Model file for the job. Use its own axes, mm. Give positions to 0.01 mm unless a question says otherwise; leave off trailing zeros. Loops run counter-clockwise (first coordinate to the right, second up) from the corner with the lowest first, then second, coordinate; pieces in that order, holes last. Notation, with made-up numbers: M -4,69.5 L 1,69.5 A20 cw 1,104.5 Z; hole C 56,6 d8. An arc over 180 degrees is marked long. Answer in a Markdown table with one row per item.
Autodesk Inventor part; units mm, degrees
ref_plane "YZ Plane" through (0, 0, 0) normal (1, 0, 0) x (0, 1, 0)
ref_plane "XZ Plane" through (0, 0, 0) normal (0, 1, 0) x (-1, 0, 0)
ref_plane "XY Plane" through (0, 0, 0) normal (0, 0, 1) x (1, 0, 0)
sketch "草圖1" plane through (0, 0, 0) normal (0, 0, 1) x (1, 0, 0)
  line L0 (-140, 0) -> (140, 0) construction
  line L1 (-140, 0) -> (140, 0) construction
  line L2 (-140, -9) -> (140, -9)
  line L3 (140, 9) -> (-140, 9)
  arc A0 (-140, 9) -> (-140, -9) centre (-140, 0) ccw
  arc A1 (140, -9) -> (140, 9) centre (140, 0) ccw
  line L4 (-140, -2.35) -> (140, -2.35) construction
  line L5 (-140, -4.5) -> (140, -4.5)
  line L6 (140, -0.2) -> (-140, -0.2)
  arc A2 (-140, -0.2) -> (-140, -4.5) centre (-140, -2.35) ccw
  arc A3 (140, -4.5) -> (140, -0.2) centre (140, -2.35) ccw
  line L7 (140, -2.35) -> (140, 0) construction
  line L8 (-140, 9) -> (-149, 9)
  line L9 (-149, 9) -> (-149, -9)
  line L10 (-149, -9) -> (-140, -9)
  line L11 (-140, -9) -> (-140, 9)
  line L12 (140, 9) -> (149, 9)
  line L13 (149, 9) -> (149, -9)
  line L14 (149, -9) -> (140, -9)
  line L15 (140, -9) -> (140, 9)
  point P0 (0, 0)
  point P1 (0, 0)
  point P2 (0, 0)
  point P3 (0, -2.35)
  point P4 (149, 0)
  point P5 (-140, -9)
  point P6 (-149, 0)
  dimension "d5" = 9
  dimension "d7" = 280
  dimension "d22" = 2.15
  dimension "d24" = 4.5
extrude "擠出1" add sketch "草圖1" along normal blind 3 contours L11 L5 L15 L2 | L10 L9 A0 | A0 L11 A2 | L15 A3 A1 | A1 L13 L14 | L9 L8 A0 | A1 L12 L13 | L3 L15 L6 L11
sketch "草圖2" plane through (0, 0, 3) normal (0, 0, 1) x (1, 0, 0)
  line L0 (-208.6, 0) -> (208.6, 0)
  line L1 (-130, -9) -> (-122, -9)
  line L2 (-122, -9) -> (-122, -12)
  line L3 (-122, -12) -> (-130, -12)
  line L4 (-130, -12) -> (-130, -9)
  line L5 (122, -9) -> (130, -9)
  line L6 (130, -9) -> (130, -12)
  line L7 (130, -12) -> (122, -12)
  line L8 (122, -12) -> (122, -9)
  arc A0 (-140, -0.2) -> (-140, -4.5) centre (-140, -2.35) ccw
  arc A1 (140, -4.5) -> (140, -0.2) centre (140, -2.35) ccw
  line L9 (-149, -9) -> (149, -9)
  point P0 (0, 0)
  point P1 (130, -10.5)
  point P2 (-130, -10.5)
  dimension "d17" = 8
  dimension "d18" = 3
  dimension "d19" = 3
  dimension "d20" = 8
  dimension "d25" = 10
  dimension "d26" = 10
extrude "擠出2" add sketch "草圖2" against normal up to surface (3 mm away)
ref_plane "工作平面2" through (-140, -2.35, 0) normal (0, 1, 0) x (1, 0, 0)
sketch "草圖4" plane through (0, 0, 3) normal (0, 0, 1) x (1, 0, 0)
  line L0 (149, 9) -> (-149, 9)
  line L1 (-149, -9) -> (-130, -9)
  line L2 (-149, 9) -> (-146, 9)
  line L3 (-146, 9) -> (-146, -9)
  line L4 (-146, -9) -> (-149, -9)
  line L5 (-149, -9) -> (-149, 9)
  line L6 (-149, 9) -> (-149, -9)
  line L7 (-149, 3) -> (-146, 3)
  line L8 (-146, 3) -> (-146, -3)
  line L9 (-146, -3) -> (-149, -3)
  line L10 (-149, -3) -> (-149, 3)
  line L11 (149, -9) -> (149, 9)
  line L12 (149, -9) -> (146, -9)
  line L13 (146, -9) -> (146, 9)
  line L14 (146, 9) -> (149, 9)
  line L15 (149, 9) -> (149, -9)
  line L16 (149, -3) -> (146, -3)
  line L17 (146, -3) -> (146, 3)
  line L18 (146, 3) -> (149, 3)
  line L19 (149, 3) -> (149, -3)
  point P0 (0, 0)
  dimension "d27" = 6
  dimension "d28" = 6
  dimension "d29" = 3
  dimension "d32" = 3
extrude "擠出3" cut sketch "草圖4" against normal up to surface (3 mm away) contours L11 L18 L13 L0 | L3 L7 L5 L0 | L11 L12 L13 L16 | L3 L1 L5 L9
sketch "草圖5" plane through (0, 0, 3) normal (0, 0, 1) x (1, 0, 0)
  arc A0 (-140, -0.2) -> (-140, -4.5) centre (-140, -2.35) ccw
  line L0 (-140, -0.2) -> (140, -0.2)
  arc A1 (140, -4.5) -> (140, -0.2) centre (140, -2.35) ccw
  line L1 (140, -4.5) -> (-140, -4.5)
  line L2 (-146, 9) -> (-146, 3)
  line L3 (-146, 3) -> (-149, 3)
  line L4 (-149, 3) -> (-149, -3)
  line L5 (-149, -3) -> (-146, -3)
  line L6 (-146, -3) -> (-146, -9)
  line L7 (-146, -9) -> (-130, -9)
  line L8 (-130, -9) -> (-130, -12)
  line L9 (-130, -12) -> (-122, -12)
  line L10 (-122, -12) -> (-122, -9)
  line L11 (-122, -9) -> (122, -9)
  line L12 (122, -9) -> (122, -12)
  line L13 (122, -12) -> (130, -12)
  line L14 (130, -12) -> (130, -9)
  line L15 (130, -9) -> (146, -9)
  line L16 (146, -9) -> (146, -3)
  line L17 (146, -3) -> (149, -3)
  line L18 (149, -3) -> (149, 3)
  line L19 (149, 3) -> (146, 3)
  line L20 (146, 3) -> (146, 9)
  line L21 (146, 9) -> (-146, 9)
  point P0 (0, 0)
equation "\"d32\" = d29"
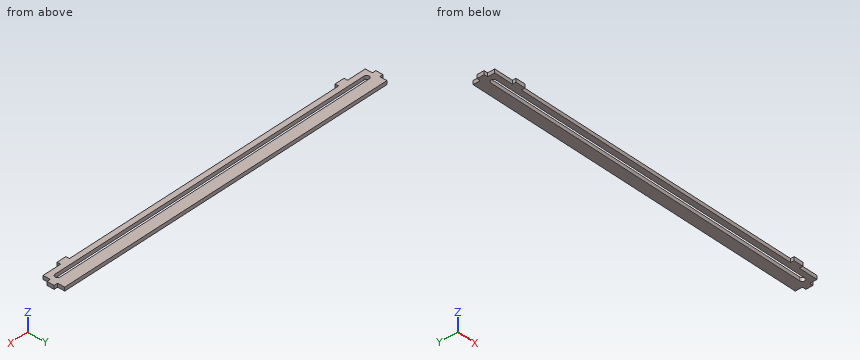
(1) Saw through at A-A, the plane x = -127.5. Give the cut face in (y, z).
Established:
| item | result |
|---|---|
| outline | M -12,0 L -4.5,0 L -4.5,3 L -12,3 Z; M -0.2,0 L 9,0 L 9,3 L -0.2,3 Z |
(2) Flat gauge pins, fed straight in: P1, Ø0.9, axis at y = 5.5, z = 2, coming from the +X side; P2, Ø1.5, axis at x = 147, z = 1, coming from the +Y side; P3, Ø0.9, axis at y = -10, z = 2, coming from the +X side. Where does each tip first touch, or does it go through?
Established:
| item | result |
|---|---|
| P1 | stops at x = 146 |
| P2 | stops at y = 3 |
| P3 | stops at x = 130 |
(3) Saw through at C-C, the plane x = 95.5. Give the cut face in (y, z).
Established:
| item | result |
|---|---|
| outline | M -9,0 L -4.5,0 L -4.5,3 L -9,3 Z; M -0.2,0 L 9,0 L 9,3 L -0.2,3 Z |
(4) Saw through at B-B, the plane z = 2.05. Give the cut face in (x, y).
Established:
| item | result |
|---|---|
| outline | M -149,-3 L -146,-3 L -146,-9 L -130,-9 L -130,-12 L -122,-12 L -122,-9 L 122,-9 L 122,-12 L 130,-12 L 130,-9 L 146,-9 L 146,-3 L 149,-3 L 149,3 L 146,3 L 146,9 L -146,9 L -146,3 L -149,3 Z; hole M -140,-4.5 L 140,-4.5 A2.15 ccw 140,-0.2 L -140,-0.2 A2.15 ccw Z |
(5) Wall check: L1, parallel to X at y = -11, z = 2.3; L2, parallel to Y at x = 7.5, z = 2.85; L3, parallel to X at y = -6.5, z = 2.25. Give the ranges that are in metal, low to high.
Established:
| item | result |
|---|---|
| L1 | x = -130 to -122, 122 to 130 |
| L2 | y = -9 to -4.5, -0.2 to 9 |
| L3 | x = -146 to 146 |
